Input: part model. Units: mm. Frame: model coordinates. Face numbers are marked on the shaded views. Coordinates: 2 decimals unless noted, no trailing zeros. Order: outer loops, then holes, each group sorted by start corner. A loop starts at its lowest first (then second) coordinate and runs counter-clockwise, first axis right, second up. Notation, with made-up numbers: (86.25, 42.5) -> (108.25, 42.5) arc R27 ccw to (108.25, 80.5) -> close; hole circle Ø8 at (-19.75, 42). An arc over 180 degrees is marked (long way). One line per item, written item: value. Start each with the question number.
from build123d import *

# Parameters (mm, degrees)
EXTRUDE1_DEPTH = 12.7


with BuildPart() as part:
    # Sketch1 → Extrude1 (new body)
    with BuildSketch(Plane.XY):
        with BuildLine():
            Line((0, 0), (76.2, 0))
            ThreePointArc((76.2, 0), (82.55, 6.35), (88.9, 0))
            Line((88.9, 0), (165.1, 0))
            Line((165.1, 0), (165.1, 38.1))
            Line((165.1, 38.1), (88.9, 38.1))
            ThreePointArc((88.9, 38.1), (82.55, 31.75), (76.2, 38.1))
            Line((76.2, 38.1), (0, 38.1))
            Line((0, 38.1), (0, 0))
        make_face()
    extrude(amount=EXTRUDE1_DEPTH)


solid = part.part
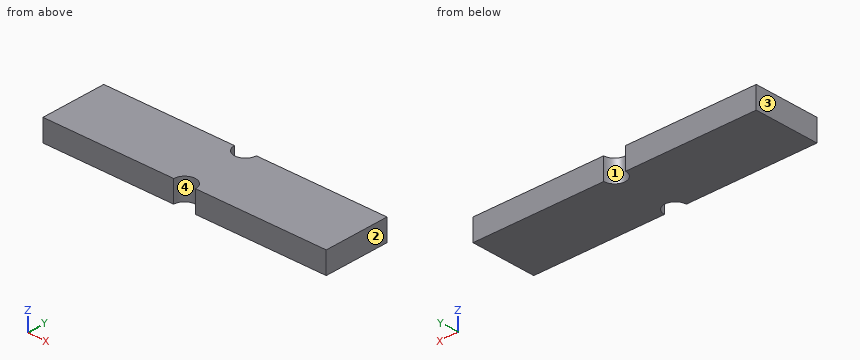
1) Section query A-A, the plane y = 4. Return the cut outline in (x, z).
2) Ray query, line 1 along X through (y, z) = (4.5, 3.25); line 2 along X through (y, z) = (3, 1). Return the intervals inside material, ascending. Write a range as from..to.
3) Section query B-B, the plane z = 2.75. Return the cut outline in (x, y), plus the area to 3 significant figures.
4) Section query C-C, the plane x = 82.55. Return the cut outline in (y, z), plus the area to 3 significant figures.
5) Mould query, pull axis X, two halves, no side actions, for the marked faces 1, 2, 3 and 4. Classes: +X half, -X half, draft (parallel to the pull), parting line (faces both ways), or undercut.
Entries:
1. outline: (0, 0) -> (77.62, 0) -> (77.62, 12.7) -> (0, 12.7) -> close; (87.48, 0) -> (165.1, 0) -> (165.1, 12.7) -> (87.48, 12.7) -> close
2. line 1: x = 0..78.07, 87.03..165.1
2. line 2: x = 0..76.95, 88.15..165.1
3. outline: (0, 0) -> (76.2, 0) arc R6.35 cw to (88.9, 0) -> (165.1, 0) -> (165.1, 38.1) -> (88.9, 38.1) arc R6.35 cw to (76.2, 38.1) -> (0, 38.1) -> close
3. area: 6,160 mm2
4. outline: (6.35, 0) -> (31.75, 0) -> (31.75, 12.7) -> (6.35, 12.7) -> close
4. area: 323 mm2
5. face 1: undercut
5. face 2: +X half
5. face 3: -X half
5. face 4: undercut
